from build123d import *

# Parameters (mm, degrees)
F0_W      = 144
F0_H      = 144
F1_DEPTH  = 25
F2_DEPTH  = 142.55
F3_T      = -2
F1_FACE_W = 144
F1_FACE_H = 144
F11_DEPTH = 5
F12_W     = 2
F12_H     = 2
F13_DEPTH = 130
F14_W     = 6
F14_H     = 144
F15_DEPTH = 10
F16_W     = 9
F16_H     = 9
F17_DEPTH = 9


with BuildPart() as f1:
    # F0 (on Top) → F1 (new body)
    with BuildSketch(Plane.XY):
        with Locations((-72, 72)):
            Rectangle(F0_W, F0_H)
    extrude(amount=F1_DEPTH)

    # F0 (on Top) → F2 (join)
    with BuildSketch(Plane.XY):
        with Locations((-72, 72)):
            Rectangle(F0_W, F0_H)
    extrude(amount=F2_DEPTH)

    # F3
    f3_openings = [f1.faces().sort_by_distance(p)[0] for p in [
        (-72, 72, 142.55),
    ]]
    offset(amount=F3_T, openings=f3_openings)

    # F1_face (on face) → F9 section 0
    with BuildSketch(Plane(origin=(-72, 72, 0), x_dir=(1, 0, 0), z_dir=(0, 0, -1))):
        Rectangle(F1_FACE_W, F1_FACE_H)
    # F8 (on 3pt) → F9 section 1
    with BuildSketch(Plane(origin=(0.0661577608, -0.0661577608, 1.8524173028), x_dir=(0.9993636652, 0.0012730747, -0.0356460925), z_dir=(-0.0356688188, 0.0356688188, -0.998726925))):
        Polygon((-2.067473366, -142.1593660309), (-2.067473366, -2.0701087697), (-142.1566169599, -2.2485664223), (-142.1566169599, -142.3378236835), align=None)
    loft()

    # F10 (on face) → F11 (cut)
    with BuildSketch(Plane.XY.offset(142.55)):
        Polygon((-142, 142), (-138, 142), (-141, 144), (-144, 144), (-144, 141), (-142, 138), align=None)
    extrude(amount=-F11_DEPTH, mode=Mode.SUBTRACT)

    # F12 (on face) → F13 (join)
    with BuildSketch(Plane.XY.offset(137.55)):
        with Locations((-140, 145)):
            Rectangle(F12_W, F12_H)
        with Locations((-145, 140)):
            Rectangle(F12_W, F12_H)
    extrude(amount=-F13_DEPTH)

    # F14 (on face) → F15 (join)
    with BuildSketch(Plane(origin=(0, 0, 0), x_dir=(1, 0, 0), z_dir=(0, 0, -1))):
        with Locations((-16, -72)):
            Rectangle(F14_W, F14_H)
        with Locations((-34.5, -72)):
            Rectangle(F14_W, F14_H)
    extrude(amount=F15_DEPTH)

    # F16 (on face) → F17 (join)
    with BuildSketch(Plane(origin=(0, 0, 0), x_dir=(1, 0, 0), z_dir=(0, 0, -1))):
        with Locations((-127.5, -127.5)):
            Rectangle(F16_W, F16_H)
        with Locations((-127.5, -16.5)):
            Rectangle(F16_W, F16_H)
    extrude(amount=F17_DEPTH)


solid = f1.part
Check sheet for the modelled part. Datum: model origin and axes. Units: mm. A direction names the side the tool comes from. Round coordinates to 2 decimals unless told otherwise and drop trailing zeros. Write each loop counter-clockwise with the first axis right and the second up, starting at its lowest first coordinate (ties: lowest second). Pieces come first, ordered by that corner, then holes. Notation, with made-up numbers: (80.25, 5) -> (131.25, 5) arc R16 cw to (131.25, 36) -> close; hole circle Ø11 at (15.5, -2.5). An arc over 180 degrees is marked (long way). Answer as CSV lines item,"result". Start each with the question number.
1) Tool access check on faces 5 (the flat face through (-25, 73, 0)), 6 (the flat face through (-142, 71, 74)), 7 (the flat face through (-132, 128, -4)), 8 (the flat face through (-128, 132, -4)). Record the directions out of +Z, -Z, +X, -X, +Y, -Y that give a thin tool (end or side, any length) a straight path to the whole face; none if there is none.
2) Go/stop test with flat-tipped pins: P1, Ø1, axis at y = 145.5, z = 92, coming from the -X side; P2, Ø5, axis at y = 54.5, z = -6.5, coming from the +X side; P3, Ø7, axis at y = 126, z = -2.5, coming from the -X side. Record where each tip stops, or that it passes through.
3) Material ranges on line 1 (Y direction, x = -68.5, z = 123.5); line 2 (X direction, y = 104.5, z = 104.5); line 3 (X direction, y = 14, z = 0.5), recorded low to high. Write a range as from..to.
4) Section check B-B on y = 18. Enter the section's corners in (x, z).
5) Release check for a two-part mould opening along X. For faces 1 (the flat face through (-19, 73, -5)), 2 (the flat face through (-123, 128, -4)), 3 (the flat face through (-132, 17, -4)), 4 (the flat face through (-128, 123, -4)) record: pulls with the +X half, pulls with the -X half, needs draft (parallel to the pull), parting line crosses it, or undercut.
6) Section check C-C on x = -68.5. Enter the section's corners in (y, z) (3 decimals).
7) Section check D-D on y = 98. Enter the section's corners in (x, z).
8) Section check A-A on z = 59.5. Enter the section's corners in (x, y).
Found:
1,face 5,"-Z, +Y, -Y"
1,face 6,"+Z"
1,face 7,"-Z, -X, +Y, -Y"
1,face 8,"-Z, -X, +Y"
2,P1,"stops at x = -141"
2,P2,"stops at x = -13"
2,P3,"stops at x = -144"
3,line 1,"y = 0..2, 142..144"
3,line 2,"x = -144..-142, -2..0"
3,line 3,"x = -144..0"
4,outline,"(-144, 0) -> (-132, 0) -> (-132, -9) -> (-123, -9) -> (-123, 0) -> (-37.5, 0) -> (-37.5, -10) -> (-31.5, -10) -> (-31.5, 0) -> (-19, 0) -> (-19, -10) -> (-13, -10) -> (-13, 0) -> (0, 0) -> (0, 142.55) -> (-2, 142.55) -> (-2, 2.57) -> (-142, 7.57) -> (-142, 142.55) -> (-144, 142.55) -> close"
5,face 1,"undercut"
5,face 2,"undercut"
5,face 3,"pulls with the -X half"
5,face 4,"needs draft"
6,outline,"(0, 0) -> (144, 0) -> (144, 142.55) -> (142, 142.55) -> (142, 9.375) -> (2, 4.375) -> (2, 142.55) -> (0, 142.55) -> close"
7,outline,"(-144, 0) -> (-37.5, 0) -> (-37.5, -10) -> (-31.5, -10) -> (-31.5, 0) -> (-19, 0) -> (-19, -10) -> (-13, -10) -> (-13, 0) -> (0, 0) -> (0, 142.55) -> (-2, 142.55) -> (-2, 5.43) -> (-142, 10.43) -> (-142, 142.55) -> (-144, 142.55) -> close"
8,outline,"(-146, 139) -> (-144, 139) -> (-144, 0) -> (0, 0) -> (0, 144) -> (-139, 144) -> (-139, 146) -> (-141, 146) -> (-141, 144) -> (-144, 144) -> (-144, 141) -> (-146, 141) -> close; hole (-142, 2) -> (-2, 2) -> (-2, 142) -> (-142, 142) -> close"
